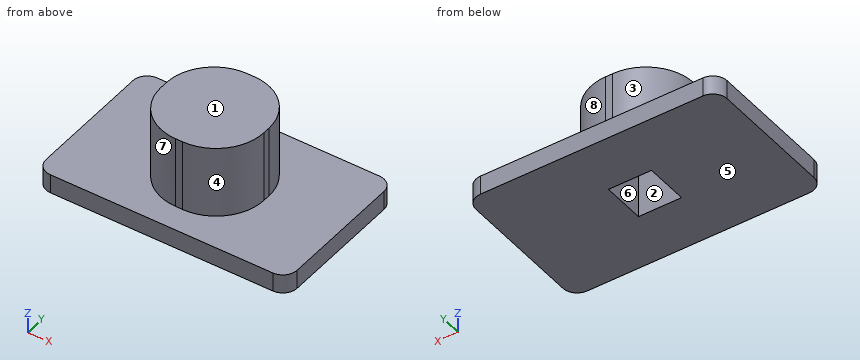
from build123d import *

# Parameters (mm, degrees)
F0_W     = 10.5
F0_H     = 6.4
F1_DEPTH = 0.8
F2_W     = 4.3
F2_H     = 4.3
F3_DEPTH = 3
F4_R     = 2
F5_R     = 0.6
F6_W     = 1.8
F6_H     = 1.8
F7_DEPTH = 2.5


with BuildPart() as f1:
    # F0 (on Top) → F1 (new body)
    with BuildSketch(Plane.XY):
        Rectangle(F0_W, F0_H)
    extrude(amount=F1_DEPTH)

    # F2 (on face) → F3 (join)
    with BuildSketch(Plane.XY.offset(0.8)):
        Rectangle(F2_W, F2_H)
    extrude(amount=F3_DEPTH)

    # F4
    f4_edges = [f1.edges().sort_by_distance(p)[0] for p in [
        (-2.15, -2.15, 2.3),
        (-2.15, 2.15, 2.3),
        (2.15, -2.15, 2.3),
        (2.15, 2.15, 2.3),
    ]]
    fillet(f4_edges, radius=F4_R)

    # F5
    f5_edges = [f1.edges().sort_by_distance(p)[0] for p in [
        (-5.25, -3.2, 0.4),
        (-5.25, 3.2, 0.4),
        (5.25, -3.2, 0.4),
        (5.25, 3.2, 0.4),
    ]]
    fillet(f5_edges, radius=F5_R)

    # F6 (on face) → F7 (cut)
    with BuildSketch(Plane(origin=(0, 0, 0), x_dir=(1, 0, 0), z_dir=(0, 0, -1))):
        Rectangle(F6_W, F6_H)
    extrude(amount=-F7_DEPTH, mode=Mode.SUBTRACT)


solid = f1.part
Can you work these out from the model? Positions are in its coordinate system, mm. Face numbers are marked on the shaded views. A direction names the side the tool comes from. Coordinates: 2 decimals unless noted, no trailing zeros. Loops run counter-clockwise (first coordinate to the right, second up) from the corner with the lowest first, then second, coordinate; pieces in that order, holes last. Notation, with made-up numbers: (44, 70.25) - (54, 70.25) arc R19 ccw to (54, 77.25) - close; hole circle Ø5 at (42, 14). An arc over 180 degrees is marked (long way). Answer as a JSON object with one key per item and string values. Group by question number.
Item 1: On a 3-axis mill with a long thin cutter (end or side, diameter ignored), from which of +Z, -Z, +X, -X, +Y, -Y can I reach the whole of each face in a straight line? I mean the marked faces 4, 5, 6, 7 and 8. Say none if no direction works.
Item 2: If we mould it in two halves opening along Y, with no side actions, what happens to the marked faces 1, 2 and 3? For each: released by +Y, released by -Y, zero draft, split by the parting line, or undercut.
Item 3: If we section it at A-A (x = -1.75): List the corners of the cut face in (y, z) for me.
Item 4: If we section it at C-C (y = 1.5): List the corners of the cut face in (x, z) for me, plus the area to 3 significant figures.
Item 5: If I drill on L1, parallel to Y at x = 0.5, z = 0.4; L2, parallel to Z at x = 3.25, y = -1.5; L3, parallel to X at y = 0.5, z = 0.5, over which ranges is the centre line in solid material (lowest first)? Write a range as from..to.
Item 6: If we section it at B-B (z = 1.05): List the corners of the cut face in (x, y) for me.
Item 7: For pin 1 (1 mm diameter, centred on x = 1.5, z = 3.5, fed in from +Y); pin 2 (0.5 mm diameter, centred on x = 0, y = -0.5, fed in from -Z), each with a flat end and sliding along its axis, tell me the tip position at first contact or that it passes through.
Item 8: If we section it at D-D (y = 0.5): List the corners of the cut face in (x, z) for me.
Returned:
{
 "1": {"face 4": "+Z, +X, -Y", "face 5": "-Z, +X, -X, +Y, -Y", "face 6": "-Z", "face 7": "+Z, -X, -Y", "face 8": "+Z, +X, +Y"},
 "2": {"face 1": "zero draft", "face 2": "undercut", "face 3": "released by +Y"},
 "3": {"outline": "(-3.2, 0) - (3.2, 0) - (3.2, 0.8) - (1.35, 0.8) - (1.35, 3.8) - (-1.35, 3.8) - (-1.35, 0.8) - (-3.2, 0.8) - close"},
 "4": {"outline": "(-5.25, 0) - (5.25, 0) - (5.25, 0.8) - (1.63, 0.8) - (1.63, 3.8) - (-1.63, 3.8) - (-1.63, 0.8) - (-5.25, 0.8) - close", "area": "18.2 mm²"},
 "5": {"L1": "y = -3.2..-0.9, 0.9..3.2", "L2": "z = 0..0.8", "L3": "x = -5.25..-0.9, 0.9..5.25"},
 "6": {"outline": "(-2.15, -0.15) arc R2 ccw to (-0.15, -2.15) - (0.15, -2.15) arc R2 ccw to (2.15, -0.15) - (2.15, 0.15) arc R2 ccw to (0.15, 2.15) - (-0.15, 2.15) arc R2 ccw to (-2.15, 0.15) - close; hole (-0.9, -0.9) - (0.9, -0.9) - (0.9, 0.9) - (-0.9, 0.9) - close"},
 "7": {"pin 1": "stops at y = 1.96", "pin 2": "stops at z = 2.5"},
 "8": {"outline": "(-5.25, 0) - (-0.9, 0) - (-0.9, 2.5) - (0.9, 2.5) - (0.9, 0) - (5.25, 0) - (5.25, 0.8) - (2.12, 0.8) - (2.12, 3.8) - (-2.12, 3.8) - (-2.12, 0.8) - (-5.25, 0.8) - close"}
}
